Here's the drawing with two shaded views (mm, measured from the low corner). I have some questions. Coordinates: 2 decimals unless noted, no trailing zeros. Write each loop counter-clockwise with the first axis right and the second up, starting at its lowest first coordinate (ties: lowest second). Pieces come first, ordered by that corner, then holes. Notation, with made-up numbers: (24.5, 14.25) - (75.5, 14.25) arc R16 ccw to (75.5, 31.25) - close; hole circle Ø1 at (56, 11.25). An arc over 180 degrees is marked (long way). Answer in a Markdown table with one row per item. Add a question column.
Item 1: Imagine slicing it at C-C (x = 16). Please give me the cut outline in (y, z).
Item 2: Imagine slicing it at A-A (y = 13). Please give me the cut outline in (x, z), plus the area to 3 significant figures.
Item 3: If I drill on probe 1 along Y at (x, z) = (50, 2.05); probe 2 along X at (y, z) = (13, 3.2), over which ranges is the centre line in solid material (lowest first)? Write a range as from..to.
Item 4: Imagine slicing it at B-B (z = 3.8). Please give me the cut outline in (x, y), plus the area to 3 significant figures.
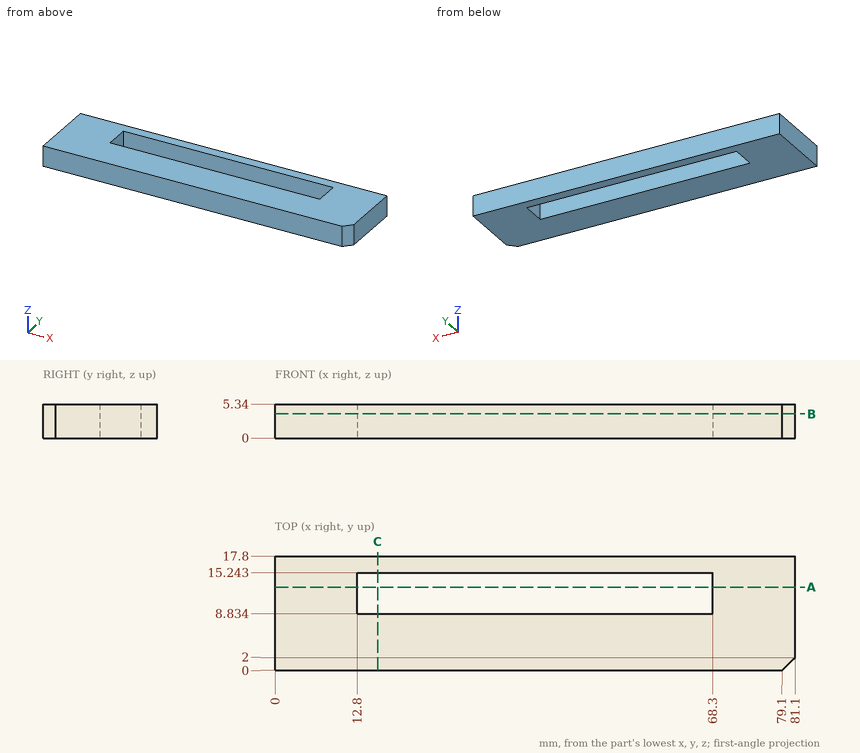
Here are the results:
| question | item | result |
|---|---|---|
| 1 | outline | (0, 0) - (8.83, 0) - (8.83, 5.34) - (0, 5.34) - close; (15.24, 0) - (17.8, 0) - (17.8, 5.34) - (15.24, 5.34) - close |
| 2 | outline | (0, 0) - (12.8, 0) - (12.8, 5.34) - (0, 5.34) - close; (68.3, 0) - (81.1, 0) - (81.1, 5.34) - (68.3, 5.34) - close |
| 2 | area | 137 mm2 |
| 3 | probe 1 | y = 0..8.83, 15.24..17.8 |
| 3 | probe 2 | x = 0..12.8, 68.3..81.1 |
| 4 | outline | (0, 0) - (79.1, 0) - (81.1, 2) - (81.1, 17.8) - (0, 17.8) - close; hole (12.8, 8.83) - (68.3, 8.83) - (68.3, 15.24) - (12.8, 15.24) - close |
| 4 | area | 1,090 mm2 |
